Geometry check sheet. Reference: the model listing, model coordinates, mm. A direction names the side the tool comes from. Coordinates: 2 decimals unless noted, no trailing zeros. Order: outer loops, then holes, each group sorted by start corner. A loop starts at its lowest first (then second) coordinate and runs counter-clockwise, first axis right, second up. Notation, with made-up numbers: (-33, 25.5) - (11, 25.5) arc R23 cw to (11, 50.5) - close; hole circle Ø8 at (-5, 44.5). An arc over 180 degrees is marked (long way). Return JSON: item names as keys, results as strings. Group by question number.
Item 1: Section check C-C on x = -7.5. Enter the section's corners in (y, z), then the cut area to 3 significant figures.
Item 2: Section check B-B on y = -1. Enter the section's corners in (x, z), then the cut area to 3 significant figures.
Item 3: Section check D-D on y = -7. Enter the section's corners in (x, z).
Item 4: Draft check along Y on faces 1 (the cylindrical face through (18, 16, 0)), 2 (the flat face through (-20, -16, 0)), 3 (the flat face through (-40, -22, 2.5)). Enter one of: pulls with the +Y half, pulls with the -Y half, needs draft (parallel to the pull), parting line crosses it, or undercut.
Item 5: Scan lines: probe 1 along Z at (x, y) = (-18, 2); probe 2 along Y at (x, z) = (-47.5, -1); probe 3 along Y at (x, z) = (35, 4.5). Record each from-to range of solid material in increasing order.
Item 6: Section check A-A on x = -37.5. Enter the section's corners in (y, z), then the cut area to 3 significant figures.
Item 7: Tool access check on faces 4 (the flat face through (-32.5, -25, 0)), 5 (the flat face through (1, -23, 0)), 6 (the flat face through (39.063, -11.74, -0.07)), 7 (the cylindrical face through (-19.962, -14.289, -18.696)). Record the directions out of +Z, -Z, +X, -X, +Y, -Y that give a thin tool (end or side, any length) a straight path to the whole face; none if there is none.
Item 8: Gauge pin test, flat ends, axial feed: pin 1 (8.5 mm diameter, centred on x = -34.5, z = -3.5, fed in from +Y); pin 2 (1.6 mm diameter, centred on y = 17, z = 0, fed in from -X); pin 3 (5 mm diameter, centred on y = -16, z = 6, fed in from +X); pin 4 (10 mm diameter, centred on y = 2, z = -12, fed in from -X). Record the tip position at first contact, or that the pin passes through.
from build123d import *

# Parameters (mm, degrees)
CROQUIS1_W                  = 105
CROQUIS1_H                  = 40
SALIENTE_EXTRUIR1_DEPTH     = 25
CORTAR_EXTRUIR1_DEPTH       = 50
CORTAR_EXTRUIR2_DEPTH       = 50
SALIENTE_EXTRUIR3_START     = -5
SALIENTE_EXTRUIR3_OUTLINE_R = 2.5
SALIENTE_EXTRUIR3_DEPTH     = 10
CORTAR_EXTRUIR3_DEPTH       = 76.208044782
REDONDEO2_R                 = 12
CORTAR_EXTRUIR4_DEPTH       = 110
CORTAR_EXTRUIR5_DEPTH       = 66
CROQUIS12_W                 = 20
CROQUIS12_H                 = 8
CROQUIS12_W_2               = 15.331196302
CROQUIS12_H_2               = 3
SALIENTE_EXTRUIR4_DEPTH     = 2.5
CROQUIS13_R                 = 1
CORTAR_EXTRUIR6_DEPTH       = 10
REDONDEO3_R                 = 2
REDONDEO4_R                 = 2
REDONDEO5_R                 = 1


# Read off the part's stored shape, not the designer's step: Saliente-Extruir3
with BuildPart() as part:
    # Croquis1 → Saliente-Extruir1 (new, symmetric)
    with BuildSketch(Plane.XY):
        Rectangle(CROQUIS1_W, CROQUIS1_H)
    extrude(amount=SALIENTE_EXTRUIR1_DEPTH, both=True)

    # Croquis2 → Cortar-Extruir1 (cut)
    with BuildSketch(Plane.XY.offset(25)):
        Polygon((-52.5, 20), (-52.5, 12), (-46.5, 12), (-26.5, 12), (-8.5, 12), (13.5, 11.241881844), (17.5, 16), (17.5, 20), align=None)
    extrude(amount=-CORTAR_EXTRUIR1_DEPTH, mode=Mode.SUBTRACT)

    # Croquis5 → Cortar-Extruir2 (cut)
    with BuildSketch(Plane.XY.offset(25)):
        with BuildLine():
            Line((52.5, 20), (17.5, 20))
            Line((17.5, 20), (25.150275796, -4.217210414))
            ThreePointArc((25.150275796, -4.217210414), (36.366474614, 13.836476048), (52.5, 0))
            Line((52.5, 0), (52.5, 20))
        make_face()
        with BuildLine():
            ThreePointArc((52.5, 0), (36.366474614, 13.836476048), (25.150275796, -4.217210414))
            ThreePointArc((25.150275796, -4.217210414), (30.224764227, -11.292496309), (38.5, -14))
            ThreePointArc((38.5, -14), (48.399494937, -9.899494937), (52.5, 0))
        make_face()
    extrude(amount=-CORTAR_EXTRUIR2_DEPTH, mode=Mode.SUBTRACT)

    # Saliente-Extruir3 outline → Saliente-Extruir3 (add)
    with BuildSketch(Plane.XY.offset(SALIENTE_EXTRUIR3_START)):
        with BuildLine():
            ThreePointArc((30.999453074, 13.78404849), (25.593027789, 10.602197019), (22.118872077, 5.378802028))
            Line((22.118872077, 5.378802028), (25.150275796, -4.217210414))
            ThreePointArc((25.150275796, -4.217210414), (28.881040119, -10.17229624), (35.035274373, -13.564500593))
            ThreePointArc((35.035274373, -13.564500593), (37.260507002, -13.415683067), (39.433873902, -12.915399918))
            Line((39.433873902, -12.915399918), (38.680800614, -10.531520596))
            ThreePointArc((38.680800614, -10.531520596), (46.18250837, 3.898461412), (31.752526362, 11.400169168))
            Line((31.752526362, 11.400169168), (30.999453074, 13.78404849))
        make_face()
        with Locations((35.216663488, 0.434324286)):
            Circle(SALIENTE_EXTRUIR3_OUTLINE_R, mode=Mode.SUBTRACT)
    extrude(amount=SALIENTE_EXTRUIR3_DEPTH)

    # Croquis8 → Cortar-Extruir3 (cut, through all)
    with BuildSketch(Plane.XY.offset(25)):
        with BuildLine():
            Line((38.5, -14), (38.5, -20))
            Line((38.5, -20), (52.5, -20))
            Line((52.5, -20), (52.5, 0))
            ThreePointArc((52.5, 0), (48.399494937, -9.899494937), (38.5, -14))
        make_face()
    extrude(amount=-CORTAR_EXTRUIR3_DEPTH, mode=Mode.SUBTRACT)

    # Redondeo2
    redondeo2_edges = [part.edges().sort_by_distance(p)[0] for p in [
        (-7, -20, -25),
        (-7, -20, 25),
    ]]
    fillet(redondeo2_edges, radius=REDONDEO2_R)

    # Croquis10 → Cortar-Extruir4 (cut)
    with BuildSketch(Plane.ZY.offset(52.5)):
        with BuildLine():
            Line((-21.966629547, 12), (-25, 12))
            Line((-25, 12), (-25, 2))
            ThreePointArc((-25, 2), (-24.22497216, 7.22497216), (-21.966629547, 12))
        make_face()
        with BuildLine():
            Line((25, 32), (-25, 32))
            Line((-25, 32), (-25, 12))
            Line((-25, 12), (-21.966629547, 12))
            ThreePointArc((-21.966629547, 12), (-15.485281374, 17.874507866), (-7, 20))
            Line((-7, 20), (7, 20))
            ThreePointArc((7, 20), (15.485281374, 17.874507866), (21.966629547, 12))
            Line((21.966629547, 12), (25, 12))
            Line((25, 12), (25, 32))
        make_face()
        with BuildLine():
            Line((25, 2), (25, 12))
            Line((25, 12), (21.966629547, 12))
            ThreePointArc((21.966629547, 12), (24.22497216, 7.22497216), (25, 2))
        make_face()
    extrude(amount=-CORTAR_EXTRUIR4_DEPTH, mode=Mode.SUBTRACT)

    # Croquis11 → Cortar-Extruir5 (cut)
    with BuildSketch(Plane.ZY.offset(52.5)):
        with BuildLine():
            Line((-20.5, 23.772379217), (20.5, 23.772379217))
            Line((20.5, 23.772379217), (20.5, -10))
            ThreePointArc((20.5, -10), (18.742640687, -14.242640687), (14.5, -16))
            Line((14.5, -16), (-14.5, -16))
            ThreePointArc((-14.5, -16), (-18.742640687, -14.242640687), (-20.5, -10))
            Line((-20.5, -10), (-20.5, 23.772379217))
        make_face()
    extrude(amount=-CORTAR_EXTRUIR5_DEPTH, mode=Mode.SUBTRACT)

    # Croquis12 → Saliente-Extruir4 (add, symmetric)
    # profile 1 of 4: a face of its own
    with BuildSketch(Plane.XY):
        with Locations((-42.5, -24)):
            Rectangle(CROQUIS12_W, CROQUIS12_H)
        with Locations((-42.5, -24.5)):
            Rectangle(CROQUIS12_W_2, CROQUIS12_H_2, mode=Mode.SUBTRACT)
    # profile 2 of 4: a face of its own
    with BuildSketch(Plane.XY):
        Polygon((11.5, -20), (-8.5, -20), (-8.5, -24), (-8.5, -28), (11.5, -28), align=None)
        with Locations((1.5, -24.5)):
            Rectangle(CROQUIS12_W_2, CROQUIS12_H_2, mode=Mode.SUBTRACT)
    # profile 3 of 4: a face of its own
    with BuildSketch(Plane.XY):
        with BuildLine():
            Line((-32.5, -20), (-32.5, -24))
            add(Edge.make_bspline(
                [(-32.5, -24), (-26.5, -20), (-20.5, -20)],
                knots=[0, 0, 0, 0.5, 0.5, 0.5], degree=2))
            Line((-20.5, -20), (-32.5, -20))
        make_face()
    # profile 4 of 4: a face of its own
    with BuildSketch(Plane.XY):
        with BuildLine():
            Line((-8.5, -20), (-20.5, -20))
            add(Edge.make_bspline(
                [(-20.5, -20), (-14.5, -20), (-8.5, -24)],
                knots=[0.5, 0.5, 0.5, 1, 1, 1], degree=2))
            Line((-8.5, -24), (-8.5, -20))
        make_face()
    extrude(amount=SALIENTE_EXTRUIR4_DEPTH, both=True)

    # Croquis13 → Cortar-Extruir6 (cut)
    with BuildSketch(Plane.ZY.offset(-17.5)):
        with Locations(Location((0, 17, 0), (0, 0, 270))):
            Circle(CROQUIS13_R)
    extrude(amount=-CORTAR_EXTRUIR6_DEPTH, mode=Mode.SUBTRACT)

    # Redondeo3
    redondeo3_edges = [part.edges().sort_by_distance(p)[0] for p in [
        (-8.5, -28, 0),
        (11.5, -28, 0),
        (-52.5, -28, 0),
        (-32.5, -28, 0),
    ]]
    fillet(redondeo3_edges, radius=REDONDEO3_R)

    # Redondeo4
    redondeo4_edges = [part.edges().sort_by_distance(p)[0] for p in [
        (11.5, -20, 0),
    ]]
    fillet(redondeo4_edges, radius=REDONDEO4_R)

    # Redondeo5
    redondeo5_edges = [part.edges().sort_by_distance(p)[0] for p in [
        (-6.165598151, -23, 0),
        (9.165598151, -23, 0),
        (9.165598151, -26, 0),
        (-6.165598151, -26, 0),
        (-50.165598151, -23, 0),
        (-34.834401849, -23, 0),
        (-34.834401849, -26, 0),
        (-50.165598151, -26, 0),
    ]]
    fillet(redondeo5_edges, radius=REDONDEO5_R)


solid = part.part
Computed:
{
 "1": {"outline": "(-27.73, -2.5) - (-20, -2.5) - (-20, -13) arc R12 ccw to (-8, -25) - (2, -25) arc R18 ccw to (11.97, -21.99) - (11.97, -20.5) - (-10, -20.5) arc R6 cw to (-16, -14.5) - (-16, 14.5) arc R6 cw to (-10, 20.5) - (11.97, 20.5) - (11.97, 21.99) arc R18 ccw to (2, 25) - (-8, 25) arc R12 ccw to (-20, 13) - (-20, 2.5) - (-27.73, 2.5) - close", "area": "425 mm²"},
 "2": {"outline": "(-52.5, -25) - (24.13, -25) - (24.13, -5) - (33.17, -5) - (33.17, 5) - (24.13, 5) - (24.13, 25) - (-52.5, 25) - (-52.5, 20.5) - (13.5, 20.5) - (13.5, -20.5) - (-52.5, -20.5) - close; (37.26, -5) - (46.63, -5) - (46.63, 5) - (37.26, 5) - close", "area": "1,310 mm²"},
 "3": {"outline": "(-52.5, -25) - (26.38, -25) - (26.38, -5) - (43.99, -5) - (43.99, 5) - (26.38, 5) - (26.38, 25) - (-52.5, 25) - (-52.5, 20.5) - (13.5, 20.5) - (13.5, -20.5) - (-52.5, -20.5) - close"},
 "4": {"face 1": "undercut", "face 2": "pulls with the +Y half", "face 3": "needs draft"},
 "5": {"probe 1": "z = -25 to -20.5, 20.5 to 25", "probe 2": "y = -28 to -26, -23 to -16", "probe 3": "y = -20 to -2.06, 2.92 to 11.93"},
 "6": {"outline": "(-28, -2.5) - (-26, -2.5) - (-26, 2.5) - (-28, 2.5) - close; (-23, -2.5) - (-20, -2.5) - (-20, -13) arc R12 ccw to (-8, -25) - (2, -25) arc R18 ccw to (12, -21.97) - (12, -20.5) - (-10, -20.5) arc R6 cw to (-16, -14.5) - (-16, 14.5) arc R6 cw to (-10, 20.5) - (12, 20.5) - (12, 21.97) arc R18 ccw to (2, 25) - (-8, 25) arc R12 ccw to (-20, 13) - (-20, 2.5) - (-23, 2.5) - close", "area": "411 mm²"},
 "7": {"face 4": "+Z, -Z, -Y", "face 5": "+Z, -Z", "face 6": "+Z, -Z, +X", "face 7": "-X, +Y"},
 "8": {"pin 1": "stops at y = -16", "pin 2": "passes through", "pin 3": "stops at x = 38.5", "pin 4": "stops at x = 13.5"}
}
